Build history of the part. All positions in model axes, mm. Face numbers are marked on the shaded views. A direction names the side the tool comes from. Coordinates: 2 decimals unless noted, no trailing zeros. Order: outer loops, then holes, each group sorted by start corner. A loop starts at its lowest first (then second) coordinate and runs counter-clockwise, first axis right, second up. Notation, with made-up numbers: M 40.25,5 L 71.25,5 A21 ccw 71.25,26 Z; hole C 13.25,66 d2. An arc over 180 degrees is marked long. Write item = value, one per line. Start each with the question number.
Q1. Pin check, flat tips, straight feed: P1, Ø11.5, axis at x = -32, z = 21, coming from the -Y side; P2, Ø14.5, axis at x = -62, z = -7, coming from the +Y side; P3, Ø10.5, axis at x = -63, z = -20, coming from the +Y side. Stop position of each tip, or through.
Q2. Band-saw the part on A-A on x = -32. Write the cut outline in (y, z).
Q3. Band-saw the part on D-D on x = 63. Write the cut outline in (y, z), plus the area to 3 significant figures.
Q4. Pull direction X, two halves, no side cores. Call the marked faces 4, 5 and 6: released by +X, released by -X, zero draft, split by the parting line, or undercut.
Q5. Band-saw the part on B-B on y = -4. Write the cut outline in (x, z).
Q6. Drill centre lines: probe 1 along X at (y, z) = (-44.75, 20); probe 2 along Z at (x, y) = (-32, 2.5); probe 3 along Z at (x, y) = (-63, -52). Where is each one in solid material? Low to high.
Q7. 3-axis set-ups, long thin cutter, end or side, ignore diameter. For the marked faces 1, 2 and 3: which of +Z, -Z, +X, -X, +Y, -Y reach the whole face in a straight line?
Q8. Band-saw the part on C-C on z = 5.5. Write the cut outline in (x, y), plus the area to 3 significant figures.
```python
from build123d import *

# Parameters (mm, degrees)
SKETCH1_W           = 106
SKETCH1_H           = 60
BOSS_EXTRUDE1_DEPTH = 10
SKETCH2_W           = 10
SKETCH2_H           = 60
BOSS_EXTRUDE2_DEPTH = 55
SKETCH3_W           = 60
SKETCH3_H           = 15
BOSS_EXTRUDE3_DEPTH = 20
SKETCH4_W           = 60
SKETCH4_H           = 15
BOSS_EXTRUDE4_DEPTH = 20
SKETCH5_R           = 4.5
CUT_EXTRUDE1_DEPTH  = 66
SKETCH6_R           = 6.5
CUT_EXTRUDE2_DEPTH  = 6.6
SKETCH7_R           = 3.3
CUT_EXTRUDE3_DEPTH  = 9.4
FILLET1_R           = 1


with BuildPart() as part:
    # Sketch1 → Boss-Extrude1 (new body)
    with BuildSketch(Plane(origin=(0, 0, 0), x_dir=(1, 0, 0), z_dir=(0, 1, 0))):
        Rectangle(SKETCH1_W, SKETCH1_H)
    extrude(amount=BOSS_EXTRUDE1_DEPTH)

    # Sketch2 → Boss-Extrude2 (add)
    with BuildSketch(Plane.XZ):
        with Locations((-48, 0)):
            Rectangle(SKETCH2_W, SKETCH2_H)
        with Locations((48, 0)):
            Rectangle(SKETCH2_W, SKETCH2_H)
    extrude(amount=BOSS_EXTRUDE2_DEPTH)

    # Sketch3 → Boss-Extrude3 (add)
    with BuildSketch(Plane(origin=(53, 0, 0), x_dir=(0, 0, -1), z_dir=(1, 0, 0))):
        with Locations((0, -47.5)):
            Rectangle(SKETCH3_W, SKETCH3_H)
    extrude(amount=BOSS_EXTRUDE3_DEPTH)

    # Sketch4 → Boss-Extrude4 (add)
    with BuildSketch(Plane.ZY.offset(53)):
        with Locations((0, -47.5)):
            Rectangle(SKETCH4_W, SKETCH4_H)
    extrude(amount=BOSS_EXTRUDE4_DEPTH)

    # Sketch5 → Cut-Extrude1 (cut, through all)
    with BuildSketch(Plane(origin=(0, 10, 0), x_dir=(1, 0, 0), z_dir=(0, 1, 0))):
        with Locations((-32, 21)):
            Circle(SKETCH5_R)
        with Locations((32, 21)):
            Circle(SKETCH5_R)
        with Locations((32, -21)):
            Circle(SKETCH5_R)
        with Locations((-32, -21)):
            Circle(SKETCH5_R)
    extrude(amount=-CUT_EXTRUDE1_DEPTH, mode=Mode.SUBTRACT)

    # Sketch6 → Cut-Extrude2 (cut)
    with BuildSketch(Plane(origin=(0, -40, 0), x_dir=(1, 0, 0), z_dir=(0, 1, 0))):
        with Locations((63, 20)):
            Circle(SKETCH6_R)
        with Locations((63, -20)):
            Circle(SKETCH6_R)
        with Locations((-63, 20)):
            Circle(SKETCH6_R)
        with Locations((-63, -20)):
            Circle(SKETCH6_R)
    extrude(amount=-CUT_EXTRUDE2_DEPTH, mode=Mode.SUBTRACT)

    # Sketch7 → Cut-Extrude3 (cut, through all)
    with BuildSketch(Plane(origin=(0, -46.6, 0), x_dir=(1, 0, 0), z_dir=(0, 1, 0))):
        with Locations((-63, 20)):
            Circle(SKETCH7_R)
        with Locations((-63, -20)):
            Circle(SKETCH7_R)
        with Locations((63, -20)):
            Circle(SKETCH7_R)
        with Locations((63, 20)):
            Circle(SKETCH7_R)
    extrude(amount=-CUT_EXTRUDE3_DEPTH, mode=Mode.SUBTRACT)

    # Fillet1
    fillet1_edges = [part.edges().sort_by_distance(p)[0] for p in [
        (-53, 10, 0),
        (0, 0, 30),
        (-43, 0, 0),
        (-43, -27.5, -30),
        (-43, -27.5, 30),
        (-58, -55, -30),
        (0, 10, 30),
        (-43, -55, 0),
        (-58, -55, 30),
        (0, 0, -30),
        (43, 0, 0),
        (43, -27.5, 30),
        (43, -27.5, -30),
        (58, -55, 30),
        (43, -55, 0),
        (58, -55, -30),
        (63, -40, 30),
        (53, -40, 0),
        (63, -40, -30),
        (73, -47.5, 30),
        (73, -55, 0),
        (73, -47.5, -30),
        (73, -40, 0),
        (53, 10, 0),
        (-63, -40, -30),
        (-53, -40, 0),
        (-63, -40, 30),
        (-73, -47.5, -30),
        (-73, -55, 0),
        (-73, -47.5, 30),
        (-73, -40, 0),
        (53, -15, 30),
        (-53, -15, 30),
        (-53, -15, -30),
        (53, -15, -30),
        (0, 10, -30),
    ]]
    fillet(fillet1_edges, radius=FILLET1_R)


solid = part.part
```
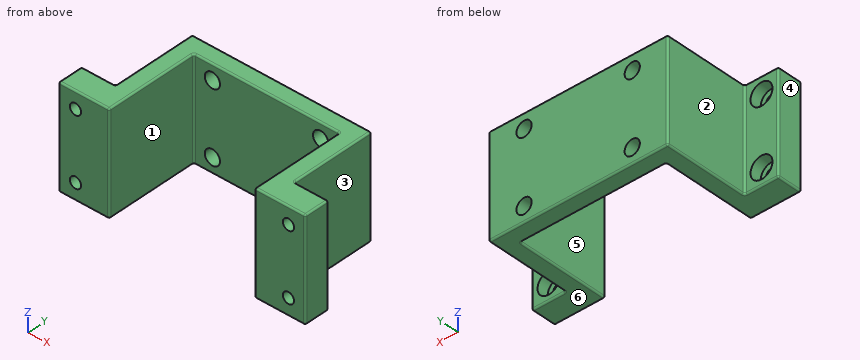
Recorded:
q1.P1 = 0
q1.P2 = -40
q1.P3 = -46.6
q2.outline = M 0,-29 A1 ccw 1,-30 L 9,-30 A1 ccw 10,-29 L 10,-25.5 L 0,-25.5 Z; M 0,-16.5 L 10,-16.5 L 10,16.5 L 0,16.5 Z; M 0,25.5 L 10,25.5 L 10,29 A1 ccw 9,30 L 1,30 A1 ccw 0,29 Z
q3.outline = M -55,-29 A1 ccw -54,-30 L -41,-30 A1 ccw -40,-29 L -40,-26.5 L -46.6,-26.5 L -46.6,-23.3 L -55,-23.3 Z; M -55,-16.7 L -46.6,-16.7 L -46.6,-13.5 L -40,-13.5 L -40,13.5 L -46.6,13.5 L -46.6,16.7 L -55,16.7 Z; M -55,23.3 L -46.6,23.3 L -46.6,26.5 L -40,26.5 L -40,29 A1 ccw -41,30 L -54,30 A1 ccw -55,29 Z
q3.area = 617 mm2
q4.face_4 = released by -X
q4.face_5 = undercut
q4.face_6 = zero draft
q5.outline = M -53,-29 A1 ccw -52,-30 L -44,-30 A1 ccw -43,-29 L -43,29 A1 ccw -44,30 L -52,30 A1 ccw -53,29 Z; M 43,-29 A1 ccw 44,-30 L 52,-30 A1 ccw 53,-29 L 53,29 A1 ccw 52,30 L 44,30 A1 ccw 43,29 Z
q6.probe_1 = -73 to -69.5, -56.5 to -43, 43 to 56.5, 69.5 to 73
q6.probe_2 = -30 to -25.5, -16.5 to 16.5, 25.5 to 30
q6.probe_3 = -30 to -23.3, -16.7 to 16.7, 23.3 to 30
q7.face_1 = +Z, -Z, -Y
q7.face_2 = +Z, -Z, -X, +Y
q7.face_3 = +Z, -Z, +X, +Y
q8.outline = M -73,-54 A1 ccw -72,-55 L -44,-55 A1 ccw -43,-54 L -43,-1 A1 cw -42,0 L 42,0 A1 cw 43,-1 L 43,-54 A1 ccw 44,-55 L 72,-55 A1 ccw 73,-54 L 73,-41 A1 ccw 72,-40 L 54,-40 A1 cw 53,-39 L 53,9 A1 ccw 52,10 L -52,10 A1 ccw -53,9 L -53,-39 A1 cw -54,-40 L -72,-40 A1 ccw -73,-41 Z
q8.area = 2,760 mm2
